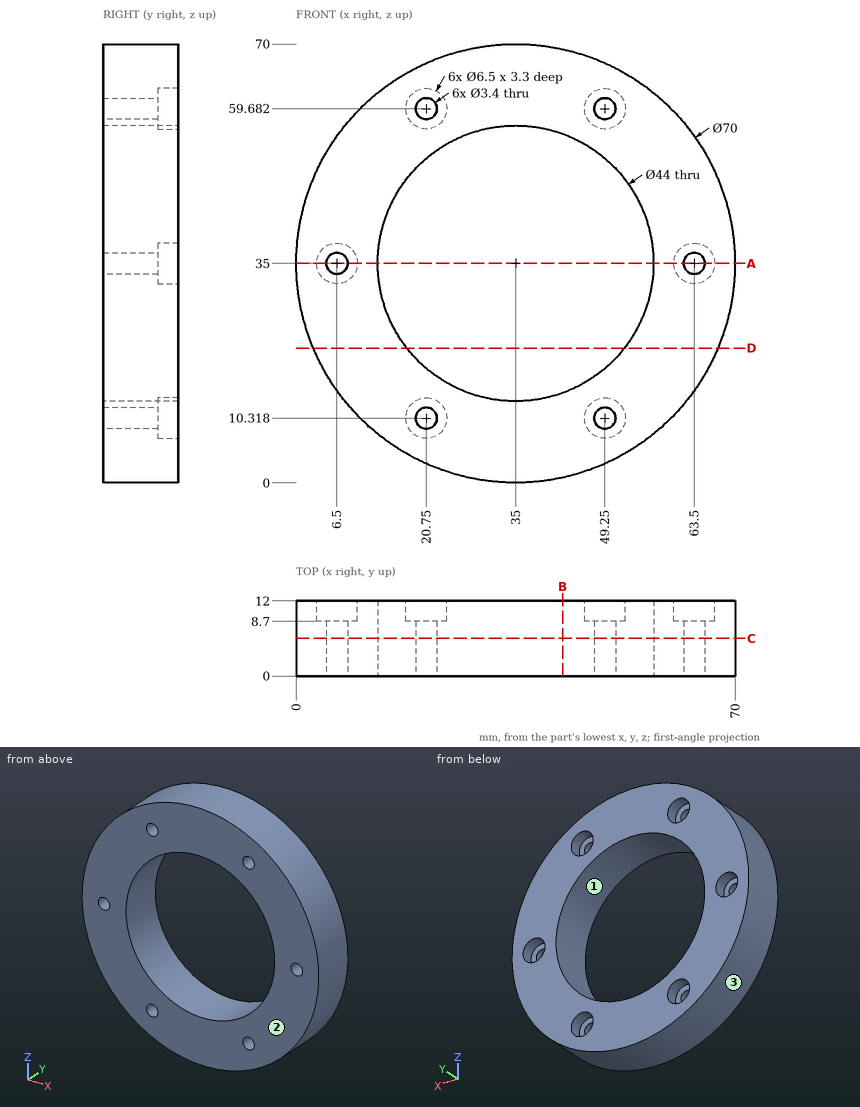
Drawing for the job (mm, zero at the part's lowest x, y, z). Coordinates: 2 decimals unless noted, no trailing zeros. Order: outer loops, then holes, each group sorted by start corner. A loop starts at its lowest first (then second) coordinate and runs counter-clockwise, first axis right, second up. Notation, with made-up numbers: (21.5, 74.25) -> (61.5, 74.25) arc R18 ccw to (61.5, 91.25) -> close; hole circle Ø2 at (53, 65.5). An arc over 180 degrees is marked (long way). Answer in a Markdown table with one row per item.
1) Band-saw the part on B-B (x = 42.5). List the corners of the cut face in (y, z), and give its area (3 significant figures).
Check values:
| item | result |
|---|---|
| outline | (0, 0.81) -> (12, 0.81) -> (12, 14.32) -> (0, 14.32) -> close; (0, 55.68) -> (12, 55.68) -> (12, 69.19) -> (0, 69.19) -> close |
| area | 324 mm2 |
2) Band-saw the part on A-A (z = 35). List the corners of the cut face in (x, y), and give its area (3 significant figures).
Check values:
| item | result |
|---|---|
| outline | (0, 0) -> (4.8, 0) -> (4.8, 8.7) -> (3.25, 8.7) -> (3.25, 12) -> (0, 12) -> close; (8.2, 0) -> (13, 0) -> (13, 12) -> (9.75, 12) -> (9.75, 8.7) -> (8.2, 8.7) -> close; (57, 0) -> (61.8, 0) -> (61.8, 8.7) -> (60.25, 8.7) -> (60.25, 12) -> (57, 12) -> close; (65.2, 0) -> (70, 0) -> (70, 12) -> (66.75, 12) -> (66.75, 8.7) -> (65.2, 8.7) -> close |
| area | 210 mm2 |
3) Mould opens along X. For the marked faces 1, 2 and 3 say: pulls with the +X half, pulls with the -X half, needs draft (parallel to the pull), parting line crosses it, or undercut.
Check values:
| item | result |
|---|---|
| face 1 | undercut |
| face 2 | needs draft |
| face 3 | parting line crosses it |
4) Drill centre lines: line 1 (X direction, y = 2.5, z = 35); line 2 (X direction, y = 3.5, z = 36) (1 decimal); line 3 (X direction, y = 2.75, z = 26) (1 decimal). Where is each one in solid material? Low to high.
Check values:
| item | result |
|---|---|
| line 1 | 0 to 4.8, 8.2 to 13, 57 to 61.8, 65.2 to 70 |
| line 2 | 0 to 5.1, 7.9 to 13, 57 to 62.1, 64.9 to 70 |
| line 3 | 1.2 to 14.9, 55.1 to 68.8 |
5) Band-saw the part on C-C (y = 6). List the corners of the cut face in (x, z).
Check values:
| item | result |
|---|---|
| outline | circle Ø70 at (35, 35); hole circle Ø3.4 at (6.5, 35); hole circle Ø44 at (35, 35); hole circle Ø3.4 at (20.75, 10.32); hole circle Ø3.4 at (20.75, 59.68); hole circle Ø3.4 at (49.25, 10.32); hole circle Ø3.4 at (49.25, 59.68); hole circle Ø3.4 at (63.5, 35) |
6) Band-saw the part on D-D (z = 21.5). List the corners of the cut face in (x, y), and give its area (3 significant figures).
Check values:
| item | result |
|---|---|
| outline | (2.71, 0) -> (17.63, 0) -> (17.63, 12) -> (2.71, 12) -> close; (52.37, 0) -> (67.29, 0) -> (67.29, 12) -> (52.37, 12) -> close |
| area | 358 mm2 |
7) Flat gauge pins, fed straight in: P1, Ø4, axis at x = 49.25, z = 10.32, coming from the +Y side; P2, Ø3, axis at x = 19, y = 8.5, coming from the +Z side (1 decimal); P3, Ø5, axis at y = 2, z = 37.5, coming from the -X side. Where does each tip first touch, or does it go through?
Check values:
| item | result |
|---|---|
| P1 | y = 8.7 |
| P2 | z = 66.9 |
| P3 | x = 0 |
